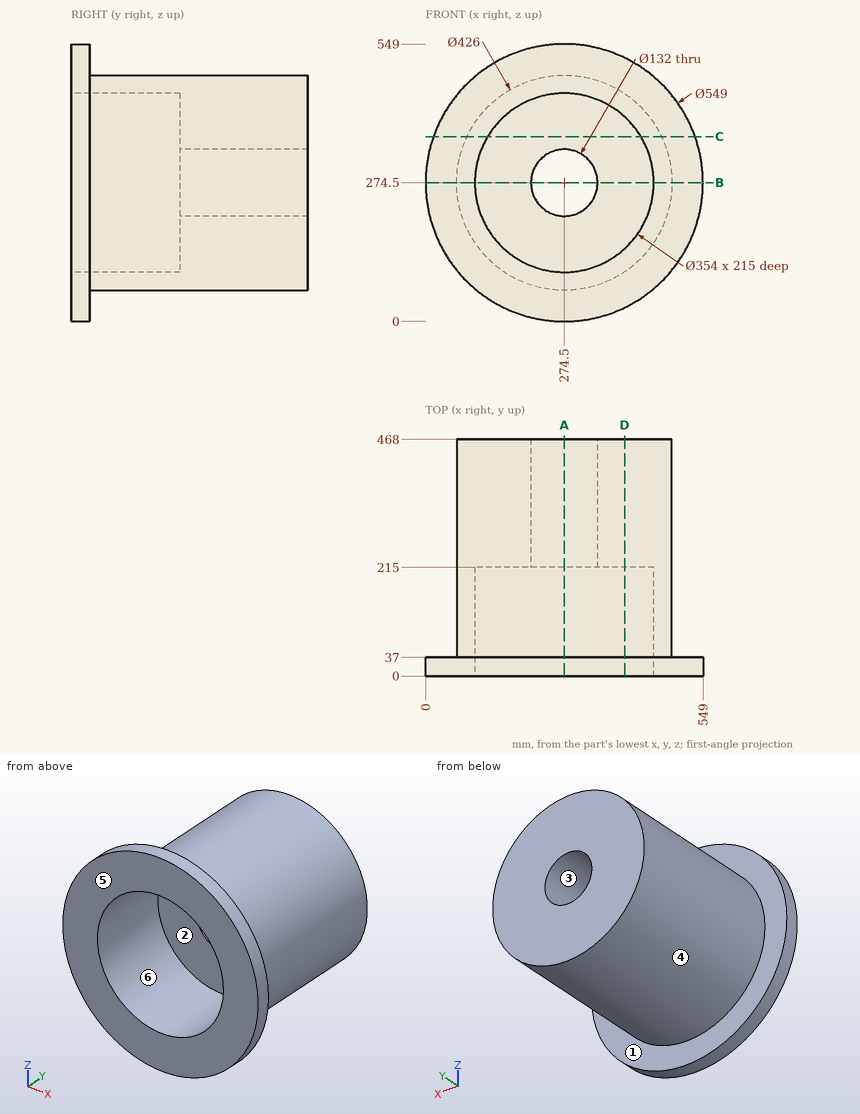
Source: three-view drawing plus pictorial views. Frame: mm from the lowest corner of the part. A direction names the side the tool comes from. Round coordinates to 2 decimals unless told otherwise and drop trailing zeros. Loops run counter-clockwise (first coordinate to the right, second up) from the corner with the lowest first, then second, coordinate; pieces in that order, holes last.
Q1. Pin query (flat end, axial travel): P1, Ø1.5, axis at x = 312, y = 343, coming from the -Z side; P2, Ø6, axis at x = 439.5, y = 53, coming from the -Z side; P3, Ø5, axis at x = 133, y = 283, coming from the -Z side; P4, Ø2, axis at x = 233.5, z = 224, coming from the +Y side. Return the tip coordinate at first contact, or that it passes through.
Q2. Section B-B on z = 274.5. Return loops of the section in (x, y).
Q3. Pull-direction query (Z, two-part tool) for the marked faces 4, 5 and 6; classes: released by +Z, released by -Z, zero draft, split by the parting line, or undercut.
Q4. Section D-D on x = 394. Return loops of the section in (y, z), plus the area to 3 significant figures.
Q5. Access query for the marked faces 1, 2 and 3. Directions: +Z, -Z, +X, -X, +Y, -Y. A direction counts if a zero-diameter tool reaches every point of the face in a straight line with its end or side. Return the directions, or none.
Q6. Section A-A on x = 274.5. Return loops of the section in (y, z), plus the area to 3 significant figures.
Q7. Material intervals for L1, parallel to X at y = 138, z = 274; L2, parallel to Y at x = 326, z = 525; L3, parallel to X at y = 183, z = 315.5, sorted ascending.
Q8. Section C-C on z = 365.5. Return loops of the section in (x, y), plus the area to 3 significant figures.
Evaluation:
1. P1: stops at z = 64.69
1. P2: stops at z = 136.21
1. P3: stops at z = 113.11
1. P4: stops at y = 468
2. outline: (0, 0) - (97.5, 0) - (97.5, 215) - (208.5, 215) - (208.5, 468) - (61.5, 468) - (61.5, 37) - (0, 37) - close; (340.5, 215) - (451.5, 215) - (451.5, 0) - (549, 0) - (549, 37) - (487.5, 37) - (487.5, 468) - (340.5, 468) - close
3. face 4: split by the parting line
3. face 5: zero draft
3. face 6: undercut
4. outline: (0, 27.38) - (37, 27.38) - (37, 98.18) - (468, 98.18) - (468, 450.82) - (37, 450.82) - (37, 521.62) - (0, 521.62) - (0, 405.07) - (215, 405.07) - (215, 143.93) - (0, 143.93) - close
4. area: 114,000 mm2
5. face 1: +Y
5. face 2: -Y
5. face 3: +Y, -Y
6. outline: (0, 0) - (37, 0) - (37, 61.5) - (468, 61.5) - (468, 208.5) - (215, 208.5) - (215, 97.5) - (0, 97.5) - close; (0, 451.5) - (215, 451.5) - (215, 340.5) - (468, 340.5) - (468, 487.5) - (37, 487.5) - (37, 549) - (0, 549) - close
6. area: 94,400 mm2
7. L1: x = 61.5 to 97.5, 451.5 to 487.5
7. L2: y = 0 to 37
7. L3: x = 65.48 to 102.31, 446.69 to 483.52
8. outline: (15.52, 0) - (122.68, 0) - (122.68, 215) - (426.32, 215) - (426.32, 0) - (533.48, 0) - (533.48, 37) - (467.08, 37) - (467.08, 468) - (81.92, 468) - (81.92, 37) - (15.52, 37) - close
8. area: 120,000 mm2
